```python
from build123d import *

# Parameters (mm, degrees)
SKETCH1_R           = 15.875
BOSS_EXTRUDE1_DEPTH = 1016
SKETCH2_R           = 34.999999977
BOSS_EXTRUDE2_DEPTH = 25.4
BOSS_EXTRUDE3_START = 25.4
SKETCH3_R           = 34.999999977
BOSS_EXTRUDE3_DEPTH = 25.4
SKETCH4_R           = 25
BOSS_EXTRUDE4_DEPTH = 254
BOSS_EXTRUDE5_START = 254
SKETCH5_R           = 25
BOSS_EXTRUDE5_DEPTH = 254
SKETCH6_R           = 17.78
CUT_EXTRUDE1_DEPTH  = 6.35
CUT_EXTRUDE2_START  = -6.35
SKETCH7_R           = 17.78
CUT_EXTRUDE2_DEPTH  = 6.35
FILLET1_R           = 2.54


with BuildPart() as part:
    # Sketch1 → Boss-Extrude1 (new body)
    with BuildSketch(Plane(origin=(0, 0, 0), x_dir=(0, 0, -1), z_dir=(1, 0, 0))):
        Circle(SKETCH1_R)
    extrude(amount=BOSS_EXTRUDE1_DEPTH)

    # Sketch2 → Boss-Extrude2 (add)
    with BuildSketch(Plane(origin=(1016, 0, 0), x_dir=(0, 0, -1), z_dir=(1, 0, 0))):
        Circle(SKETCH2_R)
    extrude(amount=BOSS_EXTRUDE2_DEPTH)

    # Sketch3 → Boss-Extrude3 (add)
    with BuildSketch(Plane.ZY.offset(BOSS_EXTRUDE3_START)):
        with Locations(Location((0, 0, 0), (0, 0, 180))):
            Circle(SKETCH3_R)
    extrude(amount=-BOSS_EXTRUDE3_DEPTH)

    # Sketch4 → Boss-Extrude4 (add)
    with BuildSketch(Plane(origin=(1041.4, 0, 0), x_dir=(0, 0, -1), z_dir=(1, 0, 0))):
        Circle(SKETCH4_R)
    extrude(amount=BOSS_EXTRUDE4_DEPTH)

    # Sketch5 → Boss-Extrude5 (add)
    with BuildSketch(Plane.ZY.offset(25.4).offset(BOSS_EXTRUDE5_START)):
        with Locations(Location((0, 0, 0), (0, 0, 180))):
            Circle(SKETCH5_R)
    extrude(amount=-BOSS_EXTRUDE5_DEPTH)

    # Sketch6 → Cut-Extrude1 (cut)
    with BuildSketch(Plane.ZY.offset(279.4)):
        Circle(SKETCH6_R)
    extrude(amount=-CUT_EXTRUDE1_DEPTH, mode=Mode.SUBTRACT)

    # Sketch7 → Cut-Extrude2 (cut)
    with BuildSketch(Plane(origin=(1295.4, 0, 0), x_dir=(0, 0, -1), z_dir=(1, 0, 0)).offset(CUT_EXTRUDE2_START)):
        with Locations(Location((0, 0, 0), (0, 0, 180))):
            Circle(SKETCH7_R)
    extrude(amount=CUT_EXTRUDE2_DEPTH, mode=Mode.SUBTRACT)

    # Fillet1
    fillet1_edges = [part.edges().sort_by_distance(p)[0] for p in [
        (-273.05, 0, -17.78),
        (1289.05, 0, -17.78),
    ]]
    fillet(fillet1_edges, radius=FILLET1_R)


solid = part.part
```
Source: CAD feature listing. Evaluate the final solid. Frame: model axes, mm. A direction names the side the tool comes from. Give positions to 0.01 mm unless a question says otherwise; leave off trailing zeros. Order: outer loops, then holes, each group sorted by start corner. A loop starts at its lowest first (then second) coordinate and runs counter-clockwise, first axis right, second up. Notation, with made-up numbers: (31.25, -26) -> (51.25, -26) arc R20 cw to (51.25, 9) -> close; hole circle Ø8 at (72, -5). An arc over 180 degrees is marked (long way). Use a Markdown table: item, result.
Q1. Pull-direction query (X, two-part tool) for faces 5 (the face through (-279.4, -6, 17)), 6 (the face through (1041.4, 8, 24)), 7 (the face through (500.888, -15.497, 3.441)); classes: +X half, -X half, draft (parallel to the pull), parting line (faces both ways), or undercut.
A:
| item | result |
|---|---|
| face 5 | -X half |
| face 6 | +X half |
| face 7 | undercut |
Q2. First-contact query: P1, Ø3, axis at x = 808, y = -15, coming from the +Z side; P2, Ø5, axis at x = -18, y = -21, coming from the +Z side; P3, Ø1.5, axis at y = 24, z = -11.5, coming from the +X side. Flat tips, straight axial feed; report the tip coordinate or a pass-through.
A:
| item | result |
|---|---|
| P1 | z = 8.35 |
| P2 | z = 29.71 |
| P3 | x = 1041.4 |
Q3. Section C-C (x = 1167.5). Return the cut outline in (y, z).
A:
| item | result |
|---|---|
| outline | circle Ø50 at (0, 0) |
Q4. Access query for faces 1 (the face through (1289.05, 0, 0)), 2 (the face through (-25.4, -8, 24)), 3 (the face through (1028.52, -31.05, -16.15)), 4 (the face through (1016, -15, -7)). Directions: +Z, -Z, +X, -X, +Y, -Y. A direction counts if a zero-diameter tool reaches every point of the face in a straight line with its end or side. Return the directions, or none.
A:
| item | result |
|---|---|
| face 1 | +X |
| face 2 | -X |
| face 3 | +X, -X |
| face 4 | none |
Q5. Section D-D (x = 847). Return the cut outline in (y, z) (3 decimals), and give its area (3 significant figures).
A:
| item | result |
|---|---|
| outline | circle Ø31.75 at (0, 0) |
| area | 792 mm^2 |
Q6. Material intervals for line 1 (Y direction, x = 1293.7, z = 0); line 2 (X direction, y = 28, z = -8); line 3 (X direction, y = 6, z = -21), sorted ascending. Write a range as [from, to].
A:
| item | result |
|---|---|
| line 1 | [-25, -17.78], [17.78, 25] |
| line 2 | [-25.4, 0], [1016, 1041.4] |
| line 3 | [-279.4, 0], [1016, 1295.4] |
